```python
from build123d import *

# Parameters (mm, degrees)
F1_DEPTH = 63.5
F0_W     = 25.4
F0_H     = 19.05
F2_DEPTH = 25.4
F3_DEPTH = 7.9375
F5_R     = 6.35
F6_DEPTH = 71.374
F7_DEPTH = 76.2
F8_R     = 12.7


with BuildPart() as f1:
    # F0 (on Front) → F1 (new body, symmetric)
    with BuildSketch(Plane.XZ):
        Polygon((41.275, -9.525), (41.275, 9.525), (22.225, 9.525), (-41.275, 9.525), (-41.275, -9.525), align=None)
    extrude(amount=F1_DEPTH, both=True)

    # F0 (on Front) → F2 (join, symmetric)
    with BuildSketch(Plane.XZ):
        with BuildLine():
            Line((22.225, 9.525), (41.275, 9.525))
            Line((41.275, 9.525), (41.275, 27.0002))
            ThreePointArc((41.275, 27.0002), (45.9246798487, 38.2255201513), (57.15, 42.8752))
            Line((57.15, 42.8752), (60.325, 42.8752))
            Line((60.325, 42.8752), (60.325, 61.9252))
            Line((60.325, 61.9252), (57.15, 61.9252))
            add(Edge.make_bspline(
                [(54.8482161911, 61.8492662184), (55.6310728691, 61.884179015), (56.3987085315, 61.9095154181), (57.15, 61.9252)],
                knots=[108.9887730241, 108.9887730241, 108.9887730241, 108.9887730241, 111.5045361635, 111.5045361635, 111.5045361635, 111.5045361635], degree=3))
            ThreePointArc((54.8482161911, 61.8492662184), (31.6534764671, 50.8682311869), (22.225, 27.0002))
            Line((22.225, 27.0002), (22.225, 9.525))
        make_face()
        with Locations((73.025, 52.4002)):
            Rectangle(F0_W, F0_H)
    extrude(amount=F2_DEPTH, both=True)

    # F0 (on Front) → F3 (join, symmetric)
    with BuildSketch(Plane.XZ):
        with BuildLine():
            Line((-41.275, 9.525), (22.225, 9.525))
            Line((22.225, 9.525), (22.225, 27.0002))
            ThreePointArc((22.225, 27.0002), (31.6534764671, 50.8682311869), (54.8482161911, 61.8492662184))
            add(Edge.make_bspline(
                [(-41.275, 9.525), (-41.5493658366, 40.8510325395), (20.933024634, 60.3367618025), (54.8482161911, 61.8492662184)],
                knots=[0, 0, 0, 0, 108.9887730241, 108.9887730241, 108.9887730241, 108.9887730241], degree=3))
        make_face()
    extrude(amount=F3_DEPTH, both=True)

    # F0 (on Front) → F4 (revolve)
    with BuildSketch(Plane.XZ):
        Polygon((85.725, 61.9252), (85.725, 42.8752), (85.725, 38.1), (111.125, 38.1), (111.125, 66.675), (85.725, 66.675), align=None)
    revolve(axis=Axis((85.725, 0, 52.3875), (0, 0, -1)))

    # F5
    f5_edges = [f1.edges().sort_by_distance(p)[0] for p in [
        (41.275, -63.5, 0),
        (-41.275, -63.5, 0),
        (41.275, 63.5, 0),
        (-41.275, 63.5, 0),
    ]]
    fillet(f5_edges, radius=F5_R)

    # F6 (add): a face of the model
    f6_faces = [f1.faces().sort_by_distance(p)[0] for p in [
        (85.725, 0, 66.675),
    ]]
    extrude(f6_faces, amount=F6_DEPTH)

    # F7 (add): a face of the model
    f7_faces = [f1.faces().sort_by_distance(p)[0] for p in [
        (-2.4929619757, -37.1068375297, 9.525),
    ]]
    extrude(f7_faces, amount=F7_DEPTH)

    # F8
    f8_edges = [f1.edges().sort_by_distance(p)[0] for p in [
        (60.325, 0, 138.049),
    ]]
    fillet(f8_edges, radius=F8_R)


solid = f1.part
```
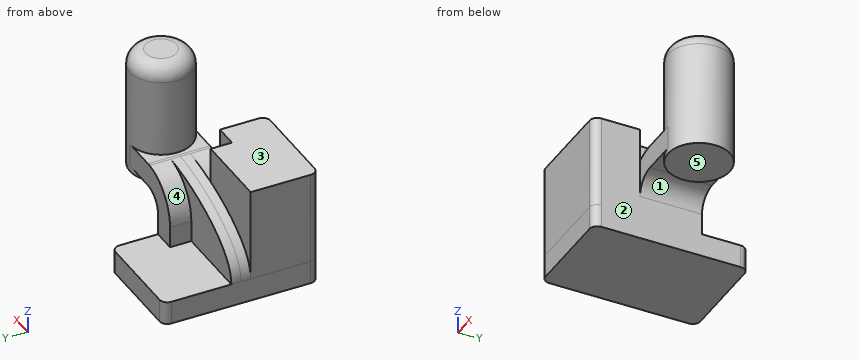
Here's how the part is built. I have some questions about the finished solid (model axes, mm). Face numbers are marked on the shaded views. A direction names the side the tool comes from. Round coordinates to 2 decimals unless told otherwise and drop trailing zeros. Order: outer loops, then holes, each group sorted by start corner. A loop starts at its lowest first (then second) coordinate and runs counter-clockwise, first axis right, second up. Notation, with made-up numbers: M 13.25,64 L 51.25,64 A36 ccw 51.25,103 Z; hole C 21.5,84.25 d5. An arc over 180 degrees is marked long. One line per question, with ' | ' between items.
1) I want a section at B-B, the plane y = 50. Write out the boundary of the cut face in (x, z) (3 decimals).
Working result:
outline: M -41.275,-9.525 L 41.275,-9.525 L 41.275,9.525 L -41.275,9.525 Z
2) For pin 1 Ø4 at (y, z) = (-15, 9.5) entering from +X (3 decimals); pin 2 Ø21 at (x, z) = (33.5, 48.5) entering from +Y; pin 3 Ø12 at (y, z) = (-20.5, 55.5) entering from +X, each with a flat end and sliding along its axis, tell me the tip position at first contact or that it passes through.
Working result:
pin 1: x = 41.275 | pin 2: y = 25.4 | pin 3: x = 106.58
3) For the marked faces 1, 2, 3, 4 and 5, which set-ups out of +Z, -Z, +X, -X, +Y, -Y let a thin tool reach every point of the face, with its end or its side?
Working result:
face 1: -Z, +Y, -Y | face 2: -Z, +X, -Y | face 3: +Z, -X, +Y, -Y | face 4: +Z, -X, +Y | face 5: -Z, +X, +Y, -Y
4) I want a section at A-A, the plane z = 97. Write out the boundary of the cut face in (x, y) (3 decimals).
Working result:
outline: C 85.725,0 d50.8
5) I need wall thicknesses on line 1 along Z through (x, y) = (78, -25); line 2 along Z through (x, y) = (-32, -8.5) (3 decimals); line 3 along Y through (x, z) = (14, 75). Which ranges of each line are inside material? Lowest first, please.
Working result:
line 1: 42.88 to 61.93 | line 2: -9.525 to 85.725 | line 3: -63.5 to -7.94
6) I want a section at C-C, the plane y = -39.5. Write out the boundary of the cut face in (x, z) (3 decimals).
Working result:
outline: M -41.275,-9.525 L 41.275,-9.525 L 41.275,85.725 L -41.275,85.725 Z
